Could you check a few things on this model? Use its own coordinates, in mm. Face numbers are marked on the shaded views. Round coordinates to 2 decimals unless told otherwise and drop trailing zeros. Write each loop counter-clockwise with the first axis right and the second up, starting at its lowest first coordinate (ties: lowest second). Pieces come first, ordered by that corner, then holes. Notation, with made-up numbers: (84.5, 18) -> (122.5, 18) arc R21 ccw to (122.5, 25) -> close; hole circle Ø9 at (64, 21.5). An arc over 180 degrees is marked (long way). Answer in a Markdown table with one row per item. Add a question column.
```python
from build123d import *

# Parameters (mm, degrees)
SKETCH1_R           = 478.75
BOSS_EXTRUDE1_DEPTH = 65
SKETCH2_R           = 456.25
SKETCH2_R_2         = 100
CUT_EXTRUDE1_DEPTH  = 35


with BuildPart() as part:
    # Sketch1 → Boss-Extrude1 (new body)
    with BuildSketch(Plane.XY):
        Circle(SKETCH1_R)
    extrude(amount=-BOSS_EXTRUDE1_DEPTH)

    # Sketch2 → Cut-Extrude1 (cut)
    with BuildSketch(Plane.XY):
        Circle(SKETCH2_R)
        Circle(SKETCH2_R_2, mode=Mode.SUBTRACT)
    extrude(amount=-CUT_EXTRUDE1_DEPTH, mode=Mode.SUBTRACT)


solid = part.part
```
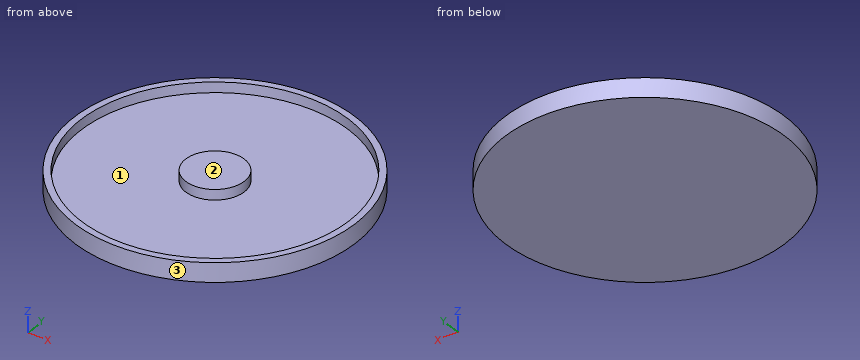
(1) Suppose I cut it at B-B, the plane z = -14. Please give me the cut outline in (x, y).
(2) I need wall thicknesses on L1, parallel to Y at x = 0, z = -15; L2, parallel to X at y = 1, z = -3.5 (3 decimals); L3, parallel to X at y = 24, z = -32. Which ranges of each line are inside material? Lowest first, please.
(3) If we mould it in two halves opening along Y, with no side actions, what happens to the marked faces 1, 2 and 3? For each: pulls with the +Y half, pulls with the -Y half, needs draft (parallel to the pull), parting line crosses it, or undercut.
(4) Suppose I cut it at A-A, the plane y = 0. Please give me the cut outline in (x, z).
(5) Suppose I cut it at D-D, the plane y = -346. Please give me the cut outline in (x, z), then the cut area to 3 significant figures.
(6) For P1, Ø12, axis at y = -355.5, z = -16, coming from the +X side; P2, Ø8, axis at y = 190.5, z = -29, coming from the -X side; P3, Ø1, axis at x = -14, y = -222, coming from the +Z side, each with a flat end and sliding along its axis, tell me the tip position at first contact or that it passes through.
Response:
| question | item | result |
|---|---|---|
| 1 | outline | circle Ø957.5 at (0, 0); circle Ø200 at (0, 0); hole circle Ø912.5 at (0, 0) |
| 2 | L1 | -478.75 to -456.25, -100 to 100, 456.25 to 478.75 |
| 2 | L2 | -478.749 to -456.249, -99.995 to 99.995, 456.249 to 478.749 |
| 2 | L3 | -478.15 to -455.62, -97.08 to 97.08, 455.62 to 478.15 |
| 3 | face 1 | undercut |
| 3 | face 2 | needs draft |
| 3 | face 3 | parting line crosses it |
| 4 | outline | (-478.75, -65) -> (478.75, -65) -> (478.75, 0) -> (456.25, 0) -> (456.25, -35) -> (100, -35) -> (100, 0) -> (-100, 0) -> (-100, -35) -> (-456.25, -35) -> (-456.25, 0) -> (-478.75, 0) -> close |
| 5 | outline | (-330.89, -65) -> (330.89, -65) -> (330.89, 0) -> (297.4, 0) -> (297.4, -35) -> (-297.4, -35) -> (-297.4, 0) -> (-330.89, 0) -> close |
| 5 | area | 22,200 mm² |
| 6 | P1 | x = 327.19 |
| 6 | P2 | x = -440.93 |
| 6 | P3 | z = -35 |
